Check sheet for the modelled part. Datum: model origin and axes. Units: mm. Face numbers are marked on the shaded views. A direction names the side the tool comes from. Give positions to 0.01 mm unless a question says otherwise; leave off trailing zeros. Order: outer loops, then holes, each group sorted by start corner. A loop starts at its lowest first (then second) coordinate and runs counter-clockwise, first axis right, second up.
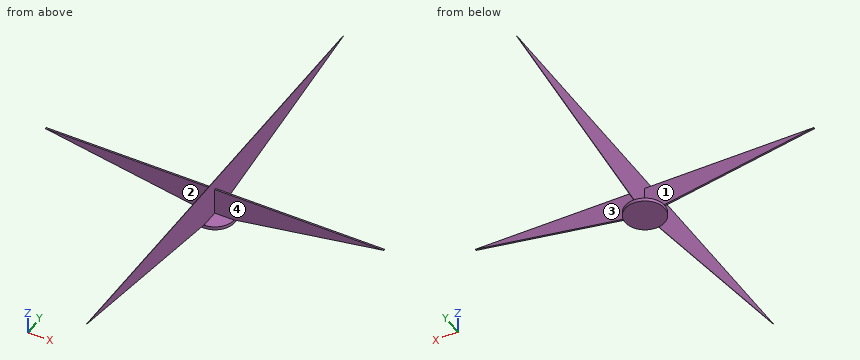
from build123d import *

# Parameters (mm, degrees)
F0_R     = 6
F1_DEPTH = 1
F3_DEPTH = 0.05
F5_DEPTH = 0.25


with BuildPart() as f1:
    # F0 (on Top) → F1 (new body)
    with BuildSketch(Plane.XY):
        Circle(F0_R)
    extrude(amount=F1_DEPTH)

    # F2 (on Right) → F3 (join, symmetric)
    with BuildSketch(Plane.YZ):
        Polygon((-68.617978, 12.099201), (0, 0), (68.617978, 12.099201), align=None)
    extrude(amount=F3_DEPTH, both=True)

    # F4 (on Front) → F5 (join, symmetric)
    with BuildSketch(Plane.XZ):
        Polygon((-51.259427, 9.03842), (0, 0), (51.259427, 9.03842), align=None)
    extrude(amount=F5_DEPTH, both=True)


solid = f1.part
1) Section check A-A, the plane z = 7.5. Record the cut outline in (x, y).
Recorded:
outline: (-42.53, -0.25) - (-0.05, -0.25) - (-0.05, -42.53) - (0.05, -42.53) - (0.05, -0.25) - (42.53, -0.25) - (42.53, 0.25) - (0.05, 0.25) - (0.05, 42.53) - (-0.05, 42.53) - (-0.05, 0.25) - (-42.53, 0.25) - close
2) Depth check by flat-ended pin: pin 1 Ø2 at (x, z) = (-1.5, 6.5) entering from -Y; pin 2 Ø3.5 at (y, z) = (-14.5, 9.5) entering from -X; pin 3 Ø2.5 at (x, z) = (30, 7) entering from +Y. Enter the tip coordinate at first touch or a pass-through.
Recorded:
pin 1: stops at y = -0.25
pin 2: stops at x = -0.05
pin 3: stops at y = 0.25
3) Section check C-C, the plane x = -12. Record the cut outline in (y, z).
Recorded:
outline: (-0.25, 2.12) - (0.25, 2.12) - (0.25, 9.04) - (-0.25, 9.04) - close
4) Material ranges on L1, parallel to Y at x = -1, z = 2.75, recorded low to high.
Recorded:
L1: y = -0.25 to 0.25
5) Section check B-B, the plane y = -39.5. Record the cut outline in (x, z).
Recorded:
outline: (-0.05, 6.96) - (0.05, 6.96) - (0.05, 12.1) - (-0.05, 12.1) - close
6) Set-up check for the marked faces 1, 2, 3 and 4: record each of +Z, -Z, +X, -X, +Y, -Y from which the full face is reachable in a straight line by a thin tool's end or side.
Recorded:
face 1: +Z, -X, +Y
face 2: +Z, -X, -Y
face 3: +Z, +X, +Y
face 4: +Z, +X, -Y
